Could you check a few things on this drawing? It's one solid part, dimensions in mm from its lowest x, y, z. Give positions to 0.01 mm unless a question says otherwise; leave off trailing zeros. Order: outer loops, then holes, each group sorted by start corner. A loop starts at its lowest first (then second) coordinate and runs counter-clockwise, first axis right, second up.
(1) Will these pins go through, and if not, where does the flat tip stop? pin 1 (18 mm diameter, centred on x = 80, z = 80, fed in from -Y); pin 2 (5 mm diameter, centred on y = 3, z = 65.5, fed in from +X); pin 3 (8.5 mm diameter, centred on x = 153.55, z = 56.45, fed in from -Y).
(2) Imagine slicing it at D-D, the plane x = 106.45. Write out the boundary of the cut face in (y, z).
(3) If we mould it in two halves opening along Z, with no side actions, what happens to the marked faces 1, 2, 3 and 4? For each: released by +Z, released by -Z, zero draft, split by the parting line, or undercut.
(4) If I drill on probe 1 along Z at (x, y) = (10, 5.5); probe 2 along Z at (x, y) = (12, 11.5); probe 3 along X at (y, z) = (1, 80.5), over which ranges is the centre line in solid material (lowest first)?
(5) Imagine slicing it at B-B, the plane x = 130. Write out the boundary of the cut face in (y, z) (3 decimals), then the cut area to 3 significant figures.
(6) Imagine slicing it at C-C, the plane y = 13. State how many separate pieces and enclosed holes the cut face has, then the cut area to 3 significant figures.
(7) Imagine slicing it at A-A, the plane z = 80. Write out the boundary of the cut face in (x, y) (3 decimals), then the cut area to 3 significant figures.
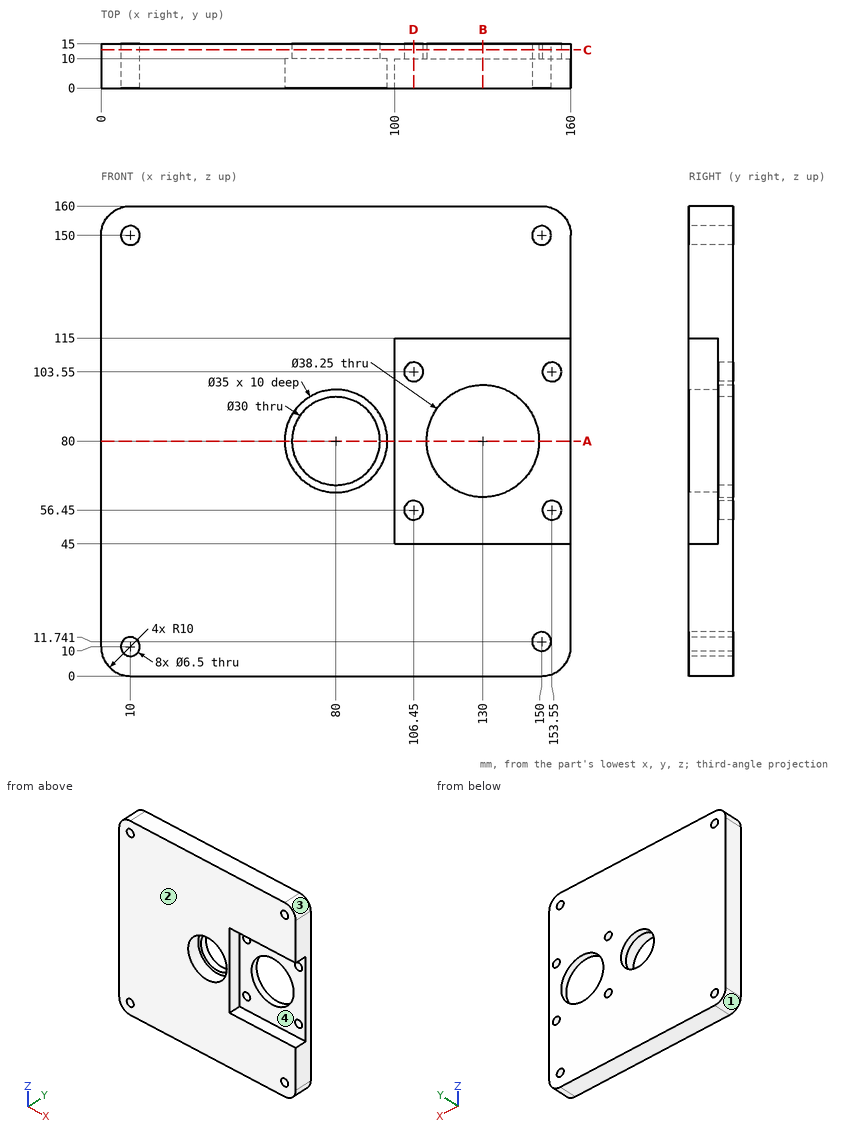
Answer block:
1. pin 1: passes through
1. pin 2: stops at x = 100
1. pin 3: stops at y = 10
2. outline: (0, 0) - (15, 0) - (15, 53.2) - (10, 53.2) - (10, 45) - (0, 45) - close; (0, 115) - (10, 115) - (10, 106.8) - (15, 106.8) - (15, 160) - (0, 160) - close; (10, 59.7) - (15, 59.7) - (15, 100.3) - (10, 100.3) - close
3. face 1: released by -Z
3. face 2: zero draft
3. face 3: released by +Z
3. face 4: undercut
4. probe 1: z = 0 to 6.75, 13.25 to 146.75, 153.25 to 160
4. probe 2: z = 0 to 7.44, 12.56 to 147.44, 152.56 to 160
4. probe 3: x = 0 to 62.51, 97.49 to 100
5. outline: (0, 0) - (15, 0) - (15, 60.875) - (10, 60.875) - (10, 45) - (0, 45) - close; (0, 115) - (10, 115) - (10, 99.125) - (15, 99.125) - (15, 160) - (0, 160) - close
5. area: 1,510 mm2
6. separate pieces: 1
6. enclosed holes: 10
6. area: 23,400 mm2
7. outline: (0, 0) - (62.5, 0) - (62.5, 10) - (65, 10) - (65, 15) - (0, 15) - close; (95, 10) - (97.5, 10) - (97.5, 0) - (100, 0) - (100, 10) - (110.875, 10) - (110.875, 15) - (95, 15) - close; (149.125, 10) - (160, 10) - (160, 15) - (149.125, 15) - close
7. area: 1,110 mm2
